Here's how the part is built. I have some questions about the finished solid (model axes, mm). A direction names the side the tool comes from. Round coordinates to 2 decimals unless told otherwise and drop trailing zeros. Loops run counter-clockwise (first coordinate to the right, second up) from the corner with the lowest first, then second, coordinate; pieces in that order, holes last. Notation, with made-up numbers: M 57.5,16 L 63.5,16 A23 ccw 63.5,33 Z; hole C 21.5,-34.75 d5. An arc over 180 degrees is marked long. Use a Markdown table: item, result.
```python
from build123d import *

# Parameters (mm, degrees)
SKETCH_1_W           = 35
SKETCH_1_H           = 45
EXTRUDE_1_DEPTH      = 13
SKETCH_2_W           = 35
SKETCH_2_H           = 90
SKETCH_2_R           = 3.6
EXTRUDE_2_DEPTH      = 7.8
SKETCH_3_W           = 35
SKETCH_3_H           = 85
EXTRUDE_3_DEPTH      = 42.2
CUT_EXTRUDE_1_DEPTH  = 65
EXTRUDE_4_DEPTH      = 17
EXTRUDE_4_DEPTH_BACK = 17
CUT_EXTRUDE_2_DEPTH  = 2.5
CUT_EXTRUDE_START    = -2.5
CUT_EXTRUDE_3_DEPTH  = 2.5
SKETCH_8_R           = 4.25
CUT_EXTRUDE_4_DEPTH  = 10
CUT_EXTRUDE_START_2  = -10
SKETCH_9_R           = 4.25
CUT_EXTRUDE_5_DEPTH  = 10


with BuildPart() as part:
    # Эскиз1 → Вытянуть1 (new body)
    with BuildSketch(Plane.XY):
        Rectangle(SKETCH_1_W, SKETCH_1_H)
    extrude(amount=EXTRUDE_1_DEPTH)

    # Эскиз2 → Вытянуть2 (add)
    with BuildSketch(Plane(origin=(0, 0, 0), x_dir=(-1, 0, 0), z_dir=(0, 0, -1))):
        Rectangle(SKETCH_2_W, SKETCH_2_H)
        with Locations((9, 35.5)):
            Circle(SKETCH_2_R, mode=Mode.SUBTRACT)
        with Locations((-9, 35.5)):
            Circle(SKETCH_2_R, mode=Mode.SUBTRACT)
        with Locations(Location((-9, -35.5, 0), (0, 0, 180))):
            Circle(SKETCH_2_R, mode=Mode.SUBTRACT)
        with Locations(Location((9, -35.5, 0), (0, 0, 180))):
            Circle(SKETCH_2_R, mode=Mode.SUBTRACT)
    extrude(amount=EXTRUDE_2_DEPTH)

    # Эскиз3 → Вытянуть3 (add)
    with BuildSketch(Plane(origin=(0, 0, -7.8), x_dir=(-1, 0, 0), z_dir=(0, 0, -1))):
        Rectangle(SKETCH_3_W, SKETCH_3_H)
    extrude(amount=EXTRUDE_3_DEPTH)

    # Эскиз4 → Вырез-Вытянуть1 (cut)
    with BuildSketch(Plane(origin=(17.5, 0, 0), x_dir=(0, 0, -1), z_dir=(1, 0, 0))):
        Polygon((72.312464651, -50.93467969), (72.312464651, 49.741254374), (44.5, 49.741254374), (44.5, 37.5), (50, 37.5), (50, 17.5), (43, 17.5), (43, -19.5), (50, -15.5), (50, -25.067494223), (47.159605794, -35), (42, -35), (42, -39.5), (50, -39.5), (50, -42.5), align=None)
    extrude(amount=-CUT_EXTRUDE_1_DEPTH, mode=Mode.SUBTRACT)

    # Эскиз5 → Вытянуть4 (add, two sides: drawn at the far end of the back side and taken through both)
    with BuildSketch(Plane(origin=(0, 0, 0), x_dir=(0, 0, -1), z_dir=(1, 0, 0)).offset(-EXTRUDE_4_DEPTH_BACK)):
        with BuildLine():
            Line((-15.487344192, -7.075529582), (-19.89829546, -11.486480851))
            Line((-19.89829546, -11.486480851), (-24.486480851, -6.89829546))
            Line((-24.486480851, -6.89829546), (-20.075529582, -2.487344192))
            ThreePointArc((-20.075529582, -2.487344192), (-7.696699141, 5.303300859), (-15.487344192, -7.075529582))
        make_face()
    extrude(amount=EXTRUDE_4_DEPTH + EXTRUDE_4_DEPTH_BACK)

    # Эскиз6 → Вырез-Вытянуть2 (cut)
    with BuildSketch(Plane(origin=(17, 0, 0), x_dir=(0, 0, -1), z_dir=(1, 0, 0))):
        with BuildLine():
            Line((-20.075529582, -2.487344192), (-24.486480851, -6.89829546))
            Line((-24.486480851, -6.89829546), (-19.89829546, -11.486480851))
            Line((-19.89829546, -11.486480851), (-15.487344192, -7.075529582))
            ThreePointArc((-15.487344192, -7.075529582), (-18.217507711, -5.217507711), (-20.075529582, -2.487344192))
        make_face()
    extrude(amount=-CUT_EXTRUDE_2_DEPTH, mode=Mode.SUBTRACT)

    # Эскиз7 → Вырез-Вытянуть3 (cut)
    with BuildSketch(Plane.ZY.offset(17).offset(CUT_EXTRUDE_START)):
        with BuildLine():
            Line((20.075529582, -2.487344192), (24.486480851, -6.89829546))
            Line((24.486480851, -6.89829546), (19.89829546, -11.486480851))
            Line((19.89829546, -11.486480851), (15.487344192, -7.075529582))
            ThreePointArc((15.487344192, -7.075529582), (18.217507711, -5.217507711), (20.075529582, -2.487344192))
        make_face()
    extrude(amount=CUT_EXTRUDE_3_DEPTH, mode=Mode.SUBTRACT)

    # Эскиз8 → Вырез-Вытянуть4 (cut)
    with BuildSketch(Plane.XZ.offset(42.5)):
        with Locations(Location((9, -36, 0), (0, 0, 270))):
            Circle(SKETCH_8_R)
        with Locations(Location((-9, -36, 0), (0, 0, 270))):
            Circle(SKETCH_8_R)
    extrude(amount=-CUT_EXTRUDE_4_DEPTH, mode=Mode.SUBTRACT)

    # Эскиз9 → Вырез-Вытянуть5 (cut)
    with BuildSketch(Plane(origin=(0, 42.5, 0), x_dir=(-1, 0, 0), z_dir=(0, 1, 0)).offset(CUT_EXTRUDE_START_2)):
        with Locations(Location((-9, -36, 0), (0, 0, 270))):
            Circle(SKETCH_9_R)
        with Locations(Location((9, -36, 0), (0, 0, 270))):
            Circle(SKETCH_9_R)
    extrude(amount=CUT_EXTRUDE_5_DEPTH, mode=Mode.SUBTRACT)


solid = part.part
```
Q1. Will these pins go through, and if not, where does the flat tip stop? P1, Ø1.2, axis at x = 5, y = -43.5, coming from the -Z side; P2, Ø11, axis at x = -7.5, y = 39, coming from the +Z side; P3, Ø6, axis at x = -1.5, y = 1.5, coming from the +Z side.
Return value:
| item | result |
|---|---|
| P1 | stops at z = -7.8 |
| P2 | stops at z = 0 |
| P3 | stops at z = 20.5 |
Q2. For faces 4 (the flat face through (9, 32.5, -36)), 5 (the flat face through (0, -44, -7.8)), 6 (the cylindrical face through (-7.065, -38.536, -3.845)), 7 (the flat face through (-0.2, -9.25, 17.66)), 8 (the cylindrical face through (-8.813, -37.57, -31.754)), which set-ups out of +Z, -Z, +X, -X, +Y, -Y let a thin tool reach every point of the face, with its end or its side?
Return value:
| item | result |
|---|---|
| face 4 | +Y |
| face 5 | -Z, +X, -X, -Y |
| face 6 | +Z |
| face 7 | +X, -X, -Y |
| face 8 | -Y |
Q3. Imagine slicing it at A-A, the plane z = -1. Please give me the cut outline in (x, y), then the cut area to 3 significant figures.
Return value:
| item | result |
|---|---|
| outline | M -17.5,-45 L 17.5,-45 L 17.5,45 L -17.5,45 Z; hole C -9,-35.5 d7.2; hole C -9,35.5 d7.2; hole C 9,-35.5 d7.2; hole C 9,35.5 d7.2 |
| area | 2,990 mm^2 |
Q4. Imagine slicing it at D-D, the plane y = 12.5. Please give me the cut outline in (x, z).
Return value:
| item | result |
|---|---|
| outline | M -17.5,-43 L 17.5,-43 L 17.5,13 L -17.5,13 Z |
Q5. Imagine slicing it at C-C, the plane z = -36. Please give me the cut outline in (x, y), then the cut area to 4 significant figures.
Return value:
| item | result |
|---|---|
| outline | M -17.5,-42.5 L -13.25,-42.5 L -13.25,-32.5 L -4.75,-32.5 L -4.75,-42.5 L 4.75,-42.5 L 4.75,-32.5 L 13.25,-32.5 L 13.25,-42.5 L 17.5,-42.5 L 17.5,42.5 L 13.25,42.5 L 13.25,32.5 L 4.75,32.5 L 4.75,42.5 L -4.75,42.5 L -4.75,32.5 L -13.25,32.5 L -13.25,42.5 L -17.5,42.5 Z |
| area | 2,635 mm^2 |
Q6. I need wall thicknesses on line 1 (Y direction, x = 9, z = -5); line 2 (X direction, y = -35.5, z = -3.75); line 3 (X direction, y = 40, z = -36). Which ranges of each line are inside material? Lowest first, please. Write a range as from..to.
Return value:
| item | result |
|---|---|
| line 1 | y = -45..-39.1, -31.9..31.9, 39.1..45 |
| line 2 | x = -17.5..-12.6, -5.4..5.4, 12.6..17.5 |
| line 3 | x = -17.5..-13.25, -4.75..4.75, 13.25..17.5 |
Q7. We'd pull the mould along Z, two halves only. Please class faces 1 (the flat face through (0.25, -29.96, -48.6)), 2 (the cylindrical face through (9.187, -37.57, -31.754)), 3 (the flat face through (0, -22.5, 6)): pulls with the +Z half, pulls with the -Z half, needs draft (parallel to the pull), parting line crosses it, or undercut.
Return value:
| item | result |
|---|---|
| face 1 | pulls with the -Z half |
| face 2 | undercut |
| face 3 | needs draft |
